The model under review builds one solid part; all positions refer to its coordinate system, in mm. Face numbers are marked on the shaded views. A direction names the side the tool comes from. Coordinates: 2 decimals unless noted, no trailing zeros. Loops run counter-clockwise (first coordinate to the right, second up) from the corner with the lowest first, then second, coordinate; pieces in that order, holes last. Notation, with made-up numbers: (83.25, 55) - (136.25, 55) arc R28 cw to (136.25, 94) - close; hole circle Ø6 at (0, 84.25). An arc over 180 degrees is marked (long way). Use a Markdown table: item, result. Add a question column.
1) Add section B-B, the plane x = -10. Give the boundary of the cut face in (y, z).
2) The part is to be moulded in two halves that separate along X. For the marked faces 4, 5 and 6, say which applies: pulls with the +X half, pulls with the -X half, needs draft (parallel to the pull), parting line crosses it, or undercut.
3) Clearance check with flat-ended pins moving along their axes: pin 1 (2.5 mm diameter, centred on x = -21, y = 0, fed in from +Z); pin 2 (0.9 mm diameter, centred on y = -14, z = 1.5, fed in from -X); pin 3 (1.3 mm diameter, centred on x = -0.5, y = 0, fed in from -Z); pin 4 (1.3 mm diameter, centred on y = 14.5, z = 4, fed in from +X). State where each tip first meets the part, or that it passes through.
4) Add section A-A, the plane z = 4. Give the boundary of the cut face in (x, y).
5) For the marked faces 1, 2 and 3, list the 3-axis set-ups (+Z, -Z, +X, -X, +Y, -Y) from which the entire face can be reached by the end or side of a thin tool; tool diameter is ignored.
6) Add section C-C, the plane y = 0. Give the number of separate pieces and of enclosed holes in the cut face, and give its area (3 significant figures).
7) To check wall thickness, follow L1, parallel to X at y = 0, z = 7; L2, parallel to X at y = 0, z = 1.4; L3, parallel to Y at x = 10, z = 1.9. State the ranges of each line that lie inside material, in increasing order. Write a range as [from, to].
8) Add section D-D, the plane z = 6.25. Give the boundary of the cut face in (x, y).
```python
from build123d import *

# Parameters (mm, degrees)
SKETCH_W        = 50
SKETCH_H        = 30
SKETCH_R        = 1.7
PAD_DEPTH       = 9
CHAMFER_SIZE    = 1.5
CHAMFER001_SIZE = 1.5
SKETCH001_R     = 2.6
SKETCH001_W     = 4.4
SKETCH001_H     = 32
SKETCH001_W_2   = 8.2
POCKET_DEPTH    = 5.5
FILLET_R        = 4
FILLET001_R     = 4
FILLET002_R     = 4
FILLET003_R     = 4
FILLET004_R     = 1
FILLET005_R     = 1
FILLET006_R     = 1
FILLET007_R     = 1
SKETCH004_R     = 3.3
PAD001_DEPTH    = 5.5


with BuildPart() as part:
    # Sketch → Pad (new body)
    with BuildSketch(Plane.XY):
        Rectangle(SKETCH_W, SKETCH_H)
        with Locations((-21, 0)):
            Circle(SKETCH_R, mode=Mode.SUBTRACT)
        with Locations((21, 0)):
            Circle(SKETCH_R, mode=Mode.SUBTRACT)
    extrude(amount=PAD_DEPTH)

    # Chamfer
    chamfer_edges = [part.edges().sort_by_distance(p)[0] for p in [
        (-22.7, 0, 9),
    ]]
    chamfer(chamfer_edges, length=CHAMFER_SIZE)

    # Chamfer001
    chamfer001_edges = [part.edges().sort_by_distance(p)[0] for p in [
        (19.3, 0, 9),
    ]]
    chamfer(chamfer001_edges, length=CHAMFER001_SIZE)

    # Sketch001 → Pocket (cut)
    with BuildSketch(Plane(origin=(0, 0, 0), x_dir=(1, 0, 0), z_dir=(0, 0, -1))):
        with Locations((-10, 0)):
            Circle(SKETCH001_R)
        with Locations((10, 0)):
            Circle(SKETCH001_R)
        Rectangle(SKETCH001_W, SKETCH001_H)
        with Locations((-21.9, 0)):
            Rectangle(SKETCH001_W_2, SKETCH001_H)
        with Locations((21.9, 0)):
            Rectangle(SKETCH001_W_2, SKETCH001_H)
    extrude(amount=-POCKET_DEPTH, mode=Mode.SUBTRACT)

    # Fillet
    fillet_edges = [part.edges().sort_by_distance(p)[0] for p in [
        (-25, -15, 7.25),
    ]]
    fillet(fillet_edges, radius=FILLET_R)

    # Fillet001
    fillet001_edges = [part.edges().sort_by_distance(p)[0] for p in [
        (-25, 15, 7.25),
    ]]
    fillet(fillet001_edges, radius=FILLET001_R)

    # Fillet002
    fillet002_edges = [part.edges().sort_by_distance(p)[0] for p in [
        (25, 15, 7.25),
    ]]
    fillet(fillet002_edges, radius=FILLET002_R)

    # Fillet003
    fillet003_edges = [part.edges().sort_by_distance(p)[0] for p in [
        (25, -15, 7.25),
    ]]
    fillet(fillet003_edges, radius=FILLET003_R)

    # Fillet004
    fillet004_edges = [part.edges().sort_by_distance(p)[0] for p in [
        (-10, 15, 0),
    ]]
    fillet(fillet004_edges, radius=FILLET004_R)

    # Fillet005
    fillet005_edges = [part.edges().sort_by_distance(p)[0] for p in [
        (10, 15, 0),
    ]]
    fillet(fillet005_edges, radius=FILLET005_R)

    # Fillet006
    fillet006_edges = [part.edges().sort_by_distance(p)[0] for p in [
        (-10, -15, 0),
    ]]
    fillet(fillet006_edges, radius=FILLET006_R)

    # Fillet007
    fillet007_edges = [part.edges().sort_by_distance(p)[0] for p in [
        (10, -15, 0),
    ]]
    fillet(fillet007_edges, radius=FILLET007_R)

    # Sketch004 → Pad001 (new body)
    with BuildSketch(Plane(origin=(0, 0, 5.5), x_dir=(1, 0, 0), z_dir=(0, 0, -1))):
        with Locations((-18, 10)):
            Circle(SKETCH004_R)
        with Locations((18, 10)):
            Circle(SKETCH004_R)
        with Locations((-18, -10)):
            Circle(SKETCH004_R)
        with Locations((18.251301, -10.165039)):
            Circle(SKETCH004_R)
    extrude(amount=PAD001_DEPTH)


solid = part.part
```
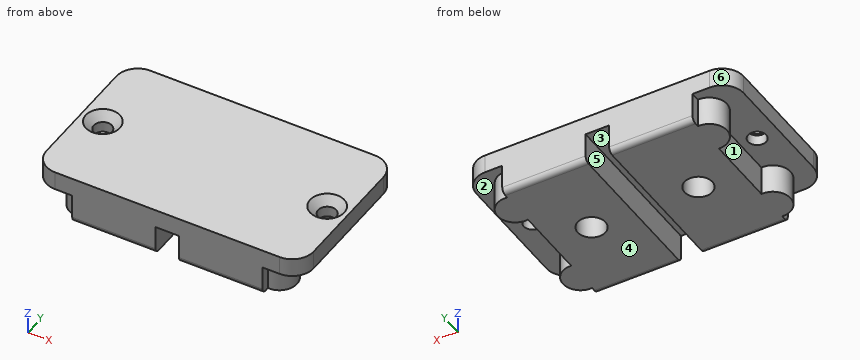
From the geometry:
| question | item | result |
|---|---|---|
| 1 | outline | (-15, 1) arc R1 ccw to (-14, 0) - (-2.6, 0) - (-2.6, 5.5) - (2.6, 5.5) - (2.6, 0) - (14, 0) arc R1 ccw to (15, 1) - (15, 9) - (-15, 9) - close |
| 2 | face 4 | needs draft |
| 2 | face 5 | undercut |
| 2 | face 6 | pulls with the -X half |
| 3 | pin 1 | passes through |
| 3 | pin 2 | stops at x = -17.8 |
| 3 | pin 3 | stops at z = 5.5 |
| 3 | pin 4 | stops at x = 17.8 |
| 4 | outline | (-17.8, -15) - (-2.2, -15) - (-2.2, 15) - (-17.8, 15) - (-17.8, 13.29) arc R3.3 ccw (long way) to (-17.8, 6.71) - (-17.8, -6.71) arc R3.3 ccw (long way) to (-17.8, -13.29) - close; (2.2, -15) - (17.8, -15) - (17.8, -13.29) arc R3.3 ccw (long way) to (17.8, -6.71) - (17.8, 6.9) arc R3.3 ccw (long way) to (17.8, 13.43) - (17.8, 15) - (2.2, 15) - close; hole circle Ø5.2 at (-10, 0); hole circle Ø5.2 at (10, 0) |
| 5 | face 1 | -Z, -X |
| 5 | face 2 | -Z, +X |
| 5 | face 3 | -Z, +Y, -Y |
| 6 | separate pieces | 3 |
| 6 | enclosed holes | 0 |
| 6 | area | 261 mm^2 |
| 7 | L1 | x = [-25, -22.7], [-19.3, 19.3], [22.7, 25] |
| 7 | L2 | x = [-17.8, -12.6], [-7.4, -2.2], [2.2, 7.4], [12.6, 17.8] |
| 7 | L3 | y = [-15, -2.6], [2.6, 15] |
| 8 | outline | (-25, -11) arc R4 ccw to (-21, -15) - (21, -15) arc R4 ccw to (25, -11) - (25, 11) arc R4 ccw to (21, 15) - (-21, 15) arc R4 ccw to (-25, 11) - close; hole circle Ø3.4 at (-21, 0); hole circle Ø3.4 at (21, 0) |
